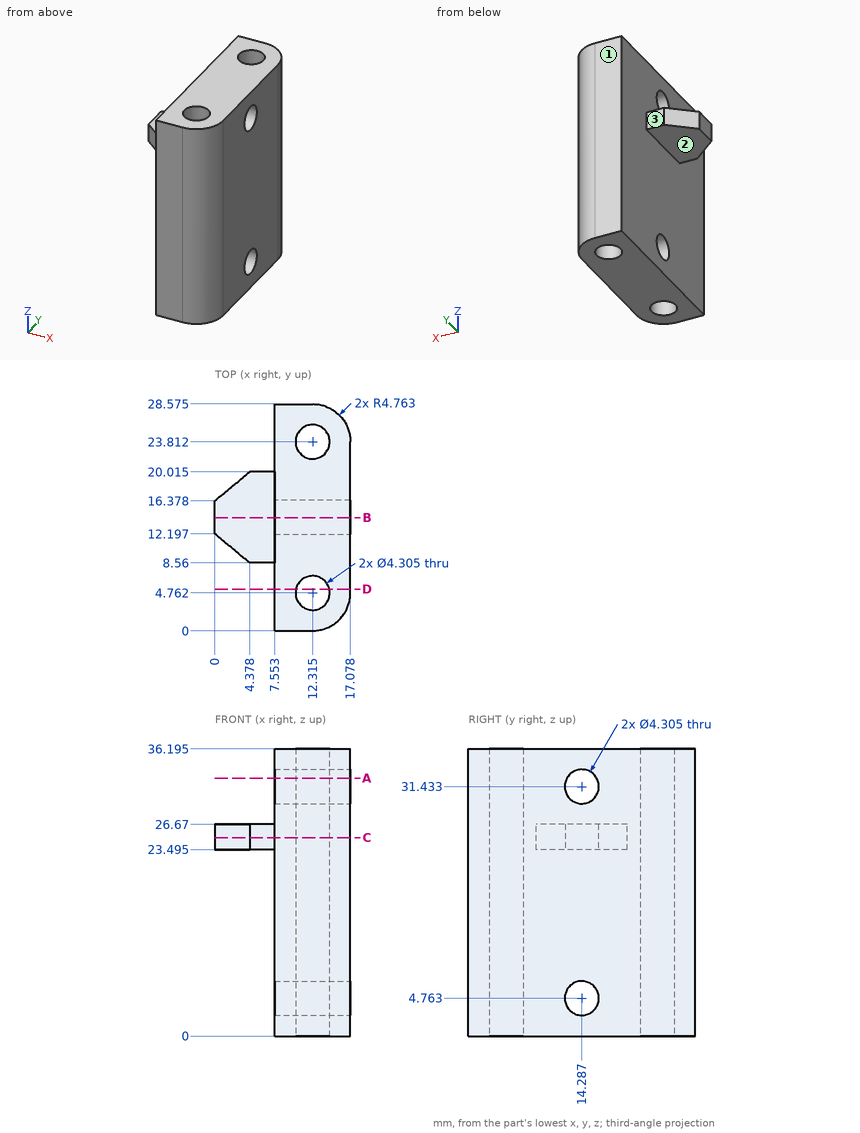
Can you work these out from the drawing? Everything is in mm from the part's minimum corner. A direction names the side the tool comes from. Coordinates: 2 decimals unless noted, no trailing zeros. Loops run counter-clockwise (first coordinate to the right, second up) from the corner with the lowest first, then second, coordinate; pieces in that order, holes last. Notation, with made-up numbers: (-10.75, -12) - (46.25, -12) arc R3 ccw to (46.25, -8) - close; hole circle Ø2 at (29, -32.75). An arc over 180 degrees is marked (long way). Use a Markdown table: item, result.
Item 1: For the marked faces 1, 2 and 3, which set-ups out of +Z, -Z, +X, -X, +Y, -Y let a thin tool reach every point of the face, with its end or its side?
Numbers:
| item | result |
|---|---|
| face 1 | +Z, -Z, +X, -X, +Y |
| face 2 | -Z, -X, +Y, -Y |
| face 3 | +Z, -Z, -X, +Y |
Item 2: I want a section at D-D on y = 5.25. Please give me the cut outline in (x, z) (1 decimal).
Numbers:
| item | result |
|---|---|
| outline | (7.6, 0) - (10.2, 0) - (10.2, 36.2) - (7.6, 36.2) - close; (14.4, 0) - (17.1, 0) - (17.1, 36.2) - (14.4, 36.2) - close |
Item 3: I want a section at B-B on y = 14.25. Please give me the cut outline in (x, z) (1 decimal), and give its area (3 significant figures).
Numbers:
| item | result |
|---|---|
| outline | (0, 23.5) - (7.6, 23.5) - (7.6, 6.9) - (17.1, 6.9) - (17.1, 29.3) - (7.6, 29.3) - (7.6, 26.7) - (0, 26.7) - close; (7.6, 0) - (17.1, 0) - (17.1, 2.6) - (7.6, 2.6) - close; (7.6, 33.6) - (17.1, 33.6) - (17.1, 36.2) - (7.6, 36.2) - close |
| area | 287 mm2 |
Item 4: Will these pins go through, and if not, where does the flat tip stop? pin 1 (4 mm diameter, centred on x = 5, y = 15, fed in from -Z) (1 decimal); pin 2 (2.5 mm diameter, centred on x = 5.5, z = 25, fed in from +Y) (1 decimal); pin 3 (3 mm diameter, centred on y = 9, z = 21.5, fed in from -X).
Numbers:
| item | result |
|---|---|
| pin 1 | stops at z = 23.5 |
| pin 2 | stops at y = 20 |
| pin 3 | stops at x = 7.55 |
Item 5: If I drill on probe 1 along Y at (x, z) = (9.5, 31.5) (1 decimal); probe 2 along Z at (x, y) = (4, 16.5) (1 decimal); probe 3 along X at (y, z) = (15.5, 12.5), over which ranges is the centre line in solid material (lowest first)? Write a range as from..to.
Numbers:
| item | result |
|---|---|
| probe 1 | y = 0..12.1, 16.4..28.6 |
| probe 2 | z = 23.5..26.7 |
| probe 3 | x = 7.55..17.08 |
Item 6: I want a section at A-A on z = 32.5. Please give me the cut outline in (x, y) (1 decimal), and give its area (3 significant figures).
Numbers:
| item | result |
|---|---|
| outline | (7.6, 0) - (12.3, 0) arc R4.8 ccw to (17.1, 4.8) - (17.1, 12.4) - (7.6, 12.4) - close; (7.6, 16.2) - (17.1, 16.2) - (17.1, 23.8) arc R4.8 ccw to (12.3, 28.6) - (7.6, 28.6) - close; hole circle Ø4.3 at (12.3, 4.8); hole circle Ø4.3 at (12.3, 23.8) |
| area | 198 mm2 |
Item 7: I want a section at C-C on z = 25. Please give me the cut outline in (x, y) (1 decimal), and give its area (3 significant figures).
Numbers:
| item | result |
|---|---|
| outline | (0, 12.2) - (4.4, 8.6) - (7.6, 8.6) - (7.6, 0) - (12.3, 0) arc R4.8 ccw to (17.1, 4.8) - (17.1, 23.8) arc R4.8 ccw to (12.3, 28.6) - (7.6, 28.6) - (7.6, 20) - (4.4, 20) - (0, 16.4) - close; hole circle Ø4.3 at (12.3, 4.8); hole circle Ø4.3 at (12.3, 23.8) |
| area | 304 mm2 |
